Design review of the part built by this model. Coordinates are the model's own, in mm. A direction names the side the tool comes from. Coordinates: 2 decimals unless noted, no trailing zeros. Write each loop counter-clockwise with the first axis right and the second up, starting at its lowest first coordinate (ties: lowest second). Pieces come first, ordered by that corner, then holes. Notation, with made-up numbers: (80, -38) -> (137, -38) arc R27 ccw to (137, -8) -> close; hole circle Ø4 at (87, -17). An arc over 180 degrees is marked (long way). Answer in a Markdown table with one row per item. Add a question column.
Item 1: Take a section at C-C, the plane y = 2. Write out the cut boundary in (x, z).
Item 2: Take a section at D-D, the plane x = 47. Give the number of separate pieces and of enclosed holes in the cut face, and give its area (3 significant figures).
Item 3: To check wall thickness, follow line 1 (Z direction, x = 47, y = -18.45); line 2 (Z direction, x = 17.2, y = 18.25); line 3 (X direction, y = -19.4, z = 17.3). State the ranges of each line that lie inside material, in increasing order.
Item 4: Take a section at B-B, the plane z = 17.3. Write out the cut boundary in (x, y).
Item 5: Draft analysis for pull direction Y (two halves, no side actions). For faces 4 (the face through (16, -17, 0)), 5 (the face through (50, 18, -17)), 6 (the face through (14, 20, 0)), state which applies: released by +Y, released by -Y, zero draft, split by the parting line, or undercut.
Item 6: Clearance check with flat-ended pins moving along their axes: P1, Ø1.5, axis at y = -19, z = 0, coming from the -X side; P2, Ø8, axis at x = 7.5, y = 11.5, coming from the +Z side (1 decimal); P3, Ø0.9, axis at x = 1.5, z = -4.5, coming from the -Y side; P4, Ø4, axis at y = 4.5, z = 15, coming from the +X side. State where each tip first meets the part, or that it passes through.
Item 7: For faces 1 (the face through (35, -19, -14.75)), 2 (the face through (3, 15, 0)), 3 (the face through (4, -19, 0)), list the 3-axis set-ups (+Z, -Z, +X, -X, +Y, -Y) from which the entire face can be reached by the end or side of a thin tool; tool diameter is ignored.
Item 8: Take a section at A-A, the plane x = 37. Write out the cut boundary in (y, z).
Autodesk Inventor part; units mm, degrees
ref_plane "YZ Plane" through (0, 0, 0) normal (1, 0, 0) x (0, 1, 0)
ref_plane "XZ Plane" through (0, 0, 0) normal (0, 1, 0) x (-1, 0, 0)
ref_plane "XY Plane" through (0, 0, 0) normal (0, 0, 1) x (1, 0, 0)
sketch "Skizze1" plane through (0, 0, 0) normal (1, 0, 0) x (0, 1, 0)
  line L0 (-20, 20) -> (20, 20)
  line L1 (20, 20) -> (20, -20)
  line L2 (20, -20) -> (-20, -20)
  line L3 (-20, -20) -> (-20, 20)
  line L4 (-20, 20) -> (20, -20) construction
  line L5 (20, 20) -> (-20, -20) construction
  point P0 (0, 0)
  dimension "d0" = 40
  dimension "d1" = 40
extrude "Extrusion1" add sketch "Skizze1" along normal blind 50
sketch "Skizze2" plane through (0, -20, 20) normal (0, 0, 1) x (1, 0, 0)
  line L0 (0, 0) -> (0, 40)
  line L1 (0, 0) -> (50, 0)
  line L2 (50, 40) -> (50, 0)
  line L3 (0, 40) -> (50, 40)
  line L4 (50, 40) -> (50, 0)
  line L5 (50, 37) -> (3, 37)
  line L6 (3, 37) -> (3, 3)
  line L7 (3, 3) -> (50, 3)
  line L8 (50, 3) -> (50, 37)
  point P0 (0, 20)
  dimension "d4" = 3
  dimension "d5" = 3
  dimension "d6" = 3
extrude "Extrusion2" cut sketch "Skizze2" against normal through all contours L7 L6 L5 L2
sketch "Skizze3" plane through (0, -20, -20) normal (0, -1, 0) x (1, 0, 0)
  line L0 (0, 0) -> (0, 40)
  line L1 (0, 0) -> (50, 0)
  line L2 (50, 40) -> (50, 0)
  line L3 (0, 40) -> (50, 40)
  line L4 (0, 20) -> (44.7617, 20) construction
  line L5 (20, 34.75) -> (50, 34.75)
  line L6 (50, 34.75) -> (50, 5.25)
  line L7 (50, 5.25) -> (20, 5.25)
  line L8 (20, 5.25) -> (20, 34.75)
  line L9 (20, 34.75) -> (50, 5.25) construction
  line L10 (50, 34.75) -> (20, 5.25) construction
  point P0 (35, 20)
  dimension "d9" = 29.5
  dimension "d10" = 30
extrude "Extrusion3" cut sketch "Skizze3" against normal blind 40 contours L7 L8 L5 L2
sketch "Skizze4" plane through (0, -20, -20) normal (0, -1, 0) x (1, 0, 0)
  line L0 (50, 5.25) -> (20, 5.25)
  line L1 (20, 5.25) -> (20, 34.75)
  line L2 (20, 34.75) -> (50, 34.75)
  line L3 (50, 40) -> (50, 34.75)
  line L4 (0, 40) -> (50, 40)
  line L5 (0, 0) -> (0, 40)
  line L6 (0, 0) -> (50, 0)
  line L7 (50, 5.25) -> (50, 0)
  line L8 (0, 20) -> (84.4351, 20) construction
  point P0 (25, 37.3)
  point P1 (25, 2.7)
  point P2 (17.2, 31)
  point P3 (17.2, 9)
  point P4 (47, 37.3)
  point P5 (47, 2.7)
  dimension "d13" = 5
  dimension "d14" = 5
  dimension "d15" = 34.6
  dimension "d16" = 17.3
  dimension "d17" = 22
  dimension "d18" = 11
  dimension "d19" = 2.8
  dimension "d20" = 2.8
  dimension "d47" = 17.3
  dimension "d48" = 17.3
  dimension "d49" = 22
  dimension "d50" = 22
hole "Bohrung1" at (25, -20, 17.3) at (25, -20, -17.3) at (17.2, -20, 11) at (17.2, -20, -11) at (47, -20, 17.3) at (47, -20, -17.3) direction (0, 1, 0) diameter 2.9 end through all
sketch "Skizze5" plane through (0, -20, -20) normal (0, -1, 0) x (1, 0, 0)
  line L0 (-4, 32.5) -> (4, 32.5)
  line L1 (4, 32.5) -> (4, 7.5)
  line L2 (4, 7.5) -> (-4, 7.5)
  line L3 (-4, 7.5) -> (-4, 32.5)
  line L4 (-4, 32.5) -> (4, 7.5) construction
  line L5 (4, 32.5) -> (-4, 7.5) construction
  circle A0 centre (17.2, 31) radius 1.45
  circle A1 centre (25, 37.3) radius 1.45
  circle A2 centre (25, 2.7) radius 1.45
  circle A3 centre (17.2, 9) radius 1.45
  line L6 (50, 5.25) -> (20, 5.25)
  line L7 (20, 5.25) -> (20, 34.75)
  line L8 (20, 34.75) -> (50, 34.75)
  line L9 (50, 40) -> (50, 34.75)
  line L10 (0, 40) -> (50, 40)
  line L11 (0, 0) -> (0, 40)
  line L12 (0, 0) -> (50, 0)
  line L13 (50, 5.25) -> (50, 0)
  point P0 (0, 20)
  dimension "d28" = 25
  dimension "d30" = 4
extrude "Extrusion4" cut sketch "Skizze5" against normal blind 33 contours L0 L11 L2 L3 | L0 L1 L2 L11
sketch "Skizze6" plane through (0, 0, 0) normal (-1, 0, 0) x (0, 0, 1)
  line L0 (0, -27.3201) -> (0, 32.8288) construction
  line L1 (-15, -12.5) -> (15, -12.5) construction
  line L2 (15, -12.5) -> (15, 4.5) construction
  line L3 (15, 4.5) -> (-15, 4.5) construction
  line L4 (-15, 4.5) -> (-15, -12.5) construction
  line L5 (-15, -12.5) -> (15, 4.5) construction
  line L6 (15, -12.5) -> (-15, 4.5) construction
  point P0 (0, 0)
  point P1 (0, -4)
  dimension "d34" = 17
  dimension "d44" = 4
  dimension "d45" = 30
hole "Bohrung2" at (0, 4.5, -15) at (0, -12.5, -15) at (0, 4.5, 15) at (0, -12.5, 15) direction (1, 0, 0) diameter 2.9 end through all
fillet "Rundung1" radius 2 2 edges at (1.5, 13, 12.5) (1.5, 13, -12.5)
equation "\"d5\" = d4"
properties part number "connection_linkFour" material "Aluminium 6061"
Answers:
| question | item | result |
|---|---|---|
| 1 | outline | (0, -20) -> (3, -20) -> (3, -12.5) -> (0, -12.5) -> close; (0, 12.5) -> (3, 12.5) -> (3, 20) -> (0, 20) -> close |
| 2 | separate pieces | 8 |
| 2 | enclosed holes | 0 |
| 2 | area | 28.2 mm^2 |
| 3 | line 1 | z = -20 to -18.75, -15.85 to -14.75, 14.75 to 15.85, 18.75 to 20 |
| 3 | line 2 | z = -20 to -12.45, -9.55 to 9.55, 12.45 to 20 |
| 3 | line 3 | x = 0 to 23.55, 26.45 to 45.55, 48.45 to 50 |
| 4 | outline | (0, -20) -> (23.55, -20) -> (23.55, -17) -> (3, -17) -> (3, 17) -> (23.55, 17) -> (23.55, 20) -> (0, 20) -> close; (26.45, -20) -> (45.55, -20) -> (45.55, -17) -> (26.45, -17) -> close; (26.45, 17) -> (45.55, 17) -> (45.55, 20) -> (26.45, 20) -> close; (48.45, -20) -> (50, -20) -> (50, -17) -> (48.45, -17) -> close; (48.45, 17) -> (50, 17) -> (50, 20) -> (48.45, 20) -> close |
| 5 | face 4 | undercut |
| 5 | face 5 | zero draft |
| 5 | face 6 | released by +Y |
| 6 | P1 | stops at x = 4 |
| 6 | P2 | passes through |
| 6 | P3 | stops at y = 13 |
| 6 | P4 | stops at x = 3 |
| 7 | face 1 | +X, +Y, -Y |
| 7 | face 2 | +Z, -Z, +X |
| 7 | face 3 | -X, -Y |
| 8 | outline | (-20, -20) -> (-17, -20) -> (-17, -14.75) -> (-20, -14.75) -> close; (-20, 14.75) -> (-17, 14.75) -> (-17, 20) -> (-20, 20) -> close; (17, -20) -> (20, -20) -> (20, -14.75) -> (17, -14.75) -> close; (17, 14.75) -> (20, 14.75) -> (20, 20) -> (17, 20) -> close |
